Geometry check sheet. Reference: the model listing, model coordinates, mm. A direction names the side the tool comes from. Round coordinates to 2 decimals unless told otherwise and drop trailing zeros. Order: outer loops, then holes, each group sorted by start corner. A loop starts at its lowest first (then second) coordinate and runs counter-clockwise, first axis right, second up.
(1) Gauge pin test, flat ends, axial feed: P1, Ø1.2, axis at y = -1387, z = 2.5, coming from the -X side; P2, Ø12, axis at x = -27.5, y = -1019.5, coming from the +Z side; P3, Ø23.5, axis at y = -350, z = 42, coming from the -X side. Record the tip position at first contact, or that the pin passes through.
(2) Thickness scan on L1, parallel to Y at x = -2.95, z = 42; L2, parallel to Z at x = -38, y = -461; L3, parallel to X at y = -94, z = 31.5. Record the ranges inside material, lowest first.
(3) Cross-section at B-B on z = 42. Enter the section's corners in (x, y), and give its area (3 significant figures).
(4) Cross-section at A-A on x = -106. Enter the section's corners in (y, z).
(5) Cross-section at C-C on y = -154.5. Enter the section's corners in (x, z).
(6) Draft check along Y on faces 1 (the face through (-59, 0, 3)), 2 (the face through (-138.026, -153.84, 1.972)), 3 (the face through (-89, -734, 4)), 4 (the face through (-59, -1489.5, 3)). Enter one of: pulls with the +Y half, pulls with the -Y half, needs draft (parallel to the pull), parting line crosses it, or undercut.
(7) Set-up check for faces 5 (the face through (-89, -734, 0)), 6 (the face through (-4, -734, 34)): record each of +Z, -Z, +X, -X, +Y, -Y from which the full face is reachable in a straight line by a thin tool's end or side.
Autodesk Inventor part; units mm, degrees
ref_plane "YZ Plane" through (0, 0, 0) normal (1, 0, 0) x (0, 1, 0)
ref_plane "XZ Plane" through (0, 0, 0) normal (0, 1, 0) x (-1, 0, 0)
ref_plane "XY Plane" through (0, 0, 0) normal (0, 0, 1) x (1, 0, 0)
sketch "Sketch1" plane through (0, 0, 0) normal (0, 0, 1) x (1, 0, 0)
  line L0 (0, 0) -> (-168.019, 0)
  line L1 (-168.019, 0) -> (-168.019, -1489.5)
  line L2 (-168.019, -1489.5) -> (0, -1489.5)
  line L3 (0, -1489.5) -> (0, 0)
  line L4 (-168.019, -1389.5) -> (-66, -1389.5)
  line L5 (-66, -1389.5) -> (-66, -1384.5)
  line L6 (-66, -1384.5) -> (-168.019, -1384.5)
  line L7 (-168.019, -1384.5) -> (-168.019, -1389.5)
  line L8 (-168.019, -892.8333) -> (-66, -892.8333)
  line L9 (-66, -892.8333) -> (-66, -887.8333)
  line L10 (-66, -887.8333) -> (-168.019, -887.8333)
  line L11 (-168.019, -887.8333) -> (-168.019, -892.8333)
  line L12 (-168.019, -396.1667) -> (-66, -396.1667)
  line L13 (-66, -396.1667) -> (-66, -391.1667)
  line L14 (-66, -391.1667) -> (-168.019, -391.1667)
  line L15 (-168.019, -391.1667) -> (-168.019, -396.1667)
  circle A0 centre (-168.019, -154.5) radius 30
  point P0 (-168.019, -396.1667)
  point P1 (-168.019, -124.5)
  point P2 (-168.019, -184.5)
  dimension "d0" = 1489.5
  dimension "d1" = 168.019
  dimension "d2" = 5
  dimension "d4" = 100
  dimension "d7" = 496.6667
  dimension "d23" = 66
  dimension "d28" = 60
  dimension "d29" = 1335
extrude "Plate1" add sketch "Sketch1" along normal blind 4 contours L3 L2 L1 L4 L5 L6 L8 L9 L10 L12 L13 L14 A0 L0
sketch "Sketch2" plane through (-4, 0, 0) normal (1, 0, 0) x (0, 1, 0)
  line L0 (-1489.5, 0) -> (0, 0)
  line L1 (0, 0) -> (0, 60)
  line L2 (0, 60) -> (-1489.5, 60)
  line L3 (-1489.5, 60) -> (-1489.5, 0)
edge flange "Flange1" height 60 angle 90 thickness 4 bend radius 4 thickness toward (1, 0, 0) relief tear relief width 4 relief depth 2 edges at (0, -744.75, 4) wall of the first edge with corners at (-4, -1489.5, 0) (-4, 0, 0) (-4, 0, 60) (-4, -1489.5, 60)
bend "Bend1"
corner "Corner1"
chamfer "Corner Chamfer1" distance 3 angle 45 6 edges at (-168.019, -1389.5, 2) (-168.019, -1384.5, 2) (-168.019, -892.8333, 2) (-168.019, -887.8333, 2) (-168.019, -391.1667, 2) (-168.019, -396.1667, 2)
sketch "Sketch4" plane through (0, -1489.5, 60) normal (1, 0, 0) x (0, 0, -1)
  line L0 (52, 0) -> (52, 1489.5) construction
  line L1 (0, 1489.5) -> (52, 1489.5) construction
  line L2 (0, 0) -> (0, 1489.5) construction
  line L3 (52, 0) -> (0, 0) construction
  circle A0 centre (18, 1139.5) radius 9
  circle A1 centre (18, 642.8333) radius 9
  circle A2 centre (18, 146.1667) radius 9
  point P0 (60, 1489.5)
  dimension "d30" = 18
  dimension "d31" = 18
  dimension "d32" = 350
  dimension "d35" = 496.6667
extrude "Cut1" cut sketch "Sketch4" against normal blind 4
equation "\"d0\" = Стрингер_длина"
equation "\"d1\" = стрингер_глубина_3"
equation "\"d2\" = паз_под_стрингер_толщина"
equation "\"d7\" = Шаг_шпангоутов"
equation "\"d23\" = паз_под_стрингер_глубина - Thickness"
equation "\"d28\" = 2 * радиус_выреза_под_сварку"
equation "\"d35\" = Шаг_шпангоутов"
equation "\"d40\" = Thickness"
equation "\"d12\" = Thickness"
equation "\"d13\" = BendReliefWidth"
equation "\"d14\" = BendReliefDepth"
equation "\"d15\" = MinimumRemnant"
equation "\"d16\" = TransitionRadius"
equation "\"d17\" = ребро_усилителей"
equation "\"d19\" = BendRadius"
equation "\"d20\" = CornerReliefSize"
equation "\"d21\" = GapSize"
equation "\"d22\" = JacobiRadiusSize"
equation "\"BendRadius\" = Thickness"
equation "\"BendReliefWidth\" = Thickness"
equation "\"BendReliefDepth\" = 0.5 * Thickness"
equation "\"CornerReliefSize\" = 4 * Thickness"
equation "\"MinimumRemnant\" = 2 * Thickness"
equation "\"TransitionRadius\" = BendRadius"
equation "\"JacobiRadiusSize\" = BendRadius"
equation "\"GapSize\" = Thickness"
properties part number "GBK 0104 stringer 3" material "Steel"
Found:
1. P1: stops at x = -66
1. P2: stops at z = 4
1. P3: stops at x = -4
2. L1: y = -1489.5 to -1352.33, -1334.33 to -855.67, -837.67 to -359, -341 to 0
2. L2: z = 0 to 4
2. L3: x = -4 to 0
3. outline: (-4, -1489.5) - (0, -1489.5) - (0, -1352.33) - (-4, -1352.33) - close; (-4, -1334.33) - (0, -1334.33) - (0, -855.67) - (-4, -855.67) - close; (-4, -837.67) - (0, -837.67) - (0, -359) - (-4, -359) - close; (-4, -341) - (0, -341) - (0, 0) - (-4, 0) - close
3. area: 5,740 mm2
4. outline: (-1489.5, 0) - (-1389.5, 0) - (-1389.5, 4) - (-1489.5, 4) - close; (-1384.5, 0) - (-892.83, 0) - (-892.83, 4) - (-1384.5, 4) - close; (-887.83, 0) - (-396.17, 0) - (-396.17, 4) - (-887.83, 4) - close; (-391.17, 0) - (0, 0) - (0, 4) - (-391.17, 4) - close
5. outline: (-138.02, 0) - (-8, 0) arc R8 ccw to (0, 8) - (0, 60) - (-4, 60) - (-4, 8) arc R4 cw to (-8, 4) - (-138.02, 4) - close
6. face 1: pulls with the +Y half
6. face 2: undercut
6. face 3: needs draft
6. face 4: pulls with the -Y half
7. face 5: -Z, +X, -X, +Y, -Y
7. face 6: +Z, -X, +Y, -Y
